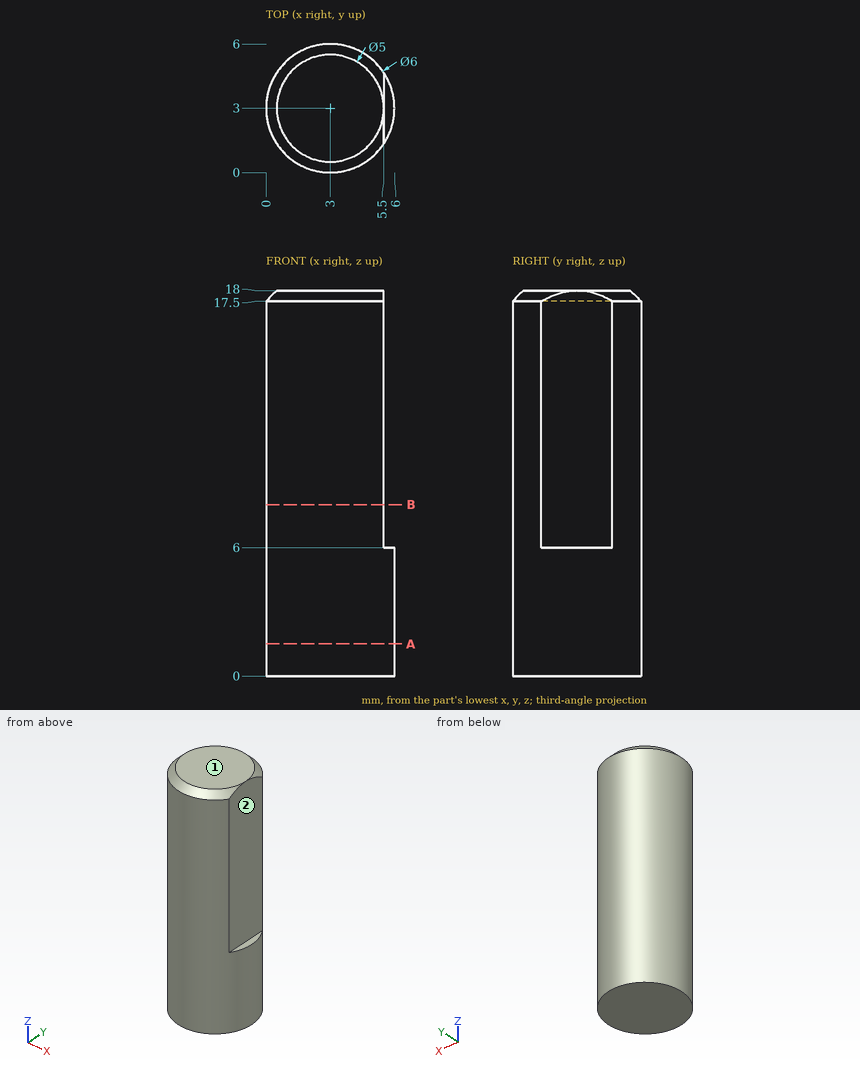
Design review of the part shown in the three views and the two pictorial views. Dimensions are in mm from the part's minimum x, y and z. A direction names the side the tool comes from. Give positions to 0.01 mm unless a question says otherwise; leave off trailing zeros. Write each loop counter-clockwise with the first axis right and the second up, starting at its lowest first coordinate (ties: lowest second). Pieces come first, ordered by that corner, then holes. Notation, with made-up numbers: (-6, 72) - (18, 72) arc R28 cw to (18, 106) - close; hole circle Ø3 at (12, 38). An arc over 180 degrees is marked (long way). Return JSON: item names as keys, results as strings. Group by question number.
(1) We need section A-A, the plane z = 1.5. Give the boundary of the cut face in (x, y), then the cut area to 3 significant figures.
(2) Machinability: for the marked faces 1 and 2, which of the approach directions +Z, -Z, +X, -X, +Y, -Y give a long, thin tool a straight path to every point of the face, cutting with its end or side? Answer none if there is none.
(3) To check wall thickness, follow probe 1 along Y at (x, z) = (5.5, 1.75); probe 2 along X at (y, z) = (2.85, 2.25); probe 3 along X at (y, z) = (3.05, 17.25). State the ranges of each line that lie inside material, in increasing order.
(4) We need section B-B, the plane z = 8. Give the boundary of the cut face in (x, y).
(5) Insertion check: pin 1 (2 mm diameter, centred on y = 1, z = 14.5, fed in from +X). The pin has a flat end and moves straight along its axis. Give the tip position at first contact, or say it passes through.
Reported:
{
 "1": {"outline": "circle Ø6 at (3, 3)", "area": "28.3 mm2"},
 "2": {"face 1": "+Z, +X, -X, +Y, -Y", "face 2": "+Z, +X, +Y, -Y"},
 "3": {"probe 1": "y = 1.34 to 4.66", "probe 2": "x = 0 to 6", "probe 3": "x = 0 to 5.5"},
 "4": {"outline": "(5.5, 1.34) - (5.5, 4.66) arc R3 ccw (long way) to start"},
 "5": {"pin 1": "stops at x = 5.5"}
}
